from build123d import *

# Parameters (mm, degrees)
SKETCH1_R           = 2.8575
BOSS_EXTRUDE1_DEPTH = 3.5052
CUT_EXTRUDE1_DEPTH  = 1.9558
SKETCH3_R           = 1.7145
BOSS_EXTRUDE2_DEPTH = 11.1125


with BuildPart() as part:
    # Sketch1 → Boss-Extrude1 (new body)
    with BuildSketch(Plane(origin=(0, 0, 0), x_dir=(1, 0, 0), z_dir=(0, 1, 0))):
        Circle(SKETCH1_R)
    extrude(amount=BOSS_EXTRUDE1_DEPTH)

    # Sketch2 → Cut-Extrude1 (cut)
    with BuildSketch(Plane.XZ):
        Polygon((1.603951217, 0), (0.801975608, 1.3890625), (-0.801975608, 1.3890625), (-1.603951217, 0), (-0.801975608, -1.3890625), (0.801975608, -1.3890625), align=None)
    extrude(amount=-CUT_EXTRUDE1_DEPTH, mode=Mode.SUBTRACT)

    # Sketch3 → Boss-Extrude2 (add)
    with BuildSketch(Plane(origin=(0, 3.5052, 0), x_dir=(1, 0, 0), z_dir=(0, 1, 0))):
        Circle(SKETCH3_R)
    extrude(amount=BOSS_EXTRUDE2_DEPTH)


solid = part.part
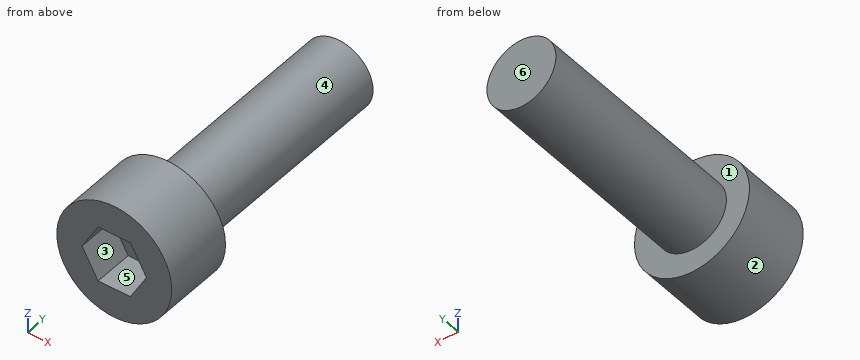
For this review, take the finished solid that the model builds, in its own axes (mm). Face numbers are marked on the shaded views. A direction names the side the tool comes from. Give positions to 0.01 mm unless a question says otherwise; leave off trailing zeros. Loops run counter-clockwise (first coordinate to the right, second up) from the corner with the lowest first, then second, coordinate; pieces in that order, holes last.
Item 1: For line 1 along Y through (x, z) = (-1, 1.45); line 2 along Y through (x, z) = (0.7, 1.3); line 3 along Z through (x, y) = (0.6, 14), list the stretches that pass through material, from the lowest coordinate up.
Item 2: Take a section at B-B, the plane y = 1. State the section outline as (x, z) points (1 decimal), and give its area (3 significant figures).
Item 3: Draft analysis for pull direction X (two halves, no side actions). For the marked faces 3, 4, 5 and 6, state which applies: +X half, -X half, draft (parallel to the pull), parting line (faces both ways), or undercut.
Item 4: Take a section at C-C, the plane z = 0.65. State the section outline as (x, y) points, and give its area (3 significant figures).
Item 5: Tool access review of the marked faces 1 and 2: name each direction out of +Z, -Z, +X, -X, +Y, -Y from which nothing blocks a thin tool from reaching the whole face with its end or side.
Item 6: Take a section at D-D, the plane y = 4.75. State the section outline as (x, z) points.
Item 7: Take a section at A-A, the plane x = 0. State the section outline as (y, z) points.
Item 8: Insertion check: pin 1 (0.8 mm diameter, centred on x = -0.5, y = 0.5, fed in from -Z); pin 2 (0.8 mm diameter, centred on x = -0.5, z = 0.5, fed in from -Y). Each pin has a flat end and moves straight along its axis. Give the tip position at first contact, or say it passes through.
Calculated:
1. line 1: y = 0 to 3.51
1. line 2: y = 1.96 to 14.62
1. line 3: z = -1.61 to 1.61
2. outline: circle Ø5.7 at (0, 0); hole (-1.6, 0) - (-0.8, -1.4) - (0.8, -1.4) - (1.6, 0) - (0.8, 1.4) - (-0.8, 1.4) - close
2. area: 19.0 mm2
3. face 3: undercut
3. face 4: parting line
3. face 5: undercut
3. face 6: draft
4. outline: (-2.78, 0) - (-1.23, 0) - (-1.23, 1.96) - (1.23, 1.96) - (1.23, 0) - (2.78, 0) - (2.78, 3.51) - (1.59, 3.51) - (1.59, 14.62) - (-1.59, 14.62) - (-1.59, 3.51) - (-2.78, 3.51) - close
4. area: 50.0 mm2
5. face 1: +Y
5. face 2: +Y, -Y
6. outline: circle Ø3.43 at (0, 0)
7. outline: (0, -2.86) - (3.51, -2.86) - (3.51, -1.71) - (14.62, -1.71) - (14.62, 1.71) - (3.51, 1.71) - (3.51, 2.86) - (0, 2.86) - (0, 1.39) - (1.96, 1.39) - (1.96, -1.39) - (0, -1.39) - close
8. pin 1: stops at z = -2.86
8. pin 2: stops at y = 1.96
